Geometry check sheet. Reference: drawing and pictorial views, mm from the part's lowest x, y, z. A direction names the side the tool comes from. Round coordinates to 2 decimals unless told otherwise and drop trailing zeros. Order: outer loops, then holes, each group sorted by start corner. A loop starts at its lowest first (then second) coordinate and runs counter-clockwise, first axis right, second up.
Q1. Depth check by flat-ended pin: P1, Ø1, axis at y = 22.5, z = 12, coming from the -X side; P2, Ø6.5, axis at x = 54, y = 13.5, coming from the -Z side; P3, Ø2.5, axis at x = 25.5, y = 27.5, coming from the +Z side; P4, Ø8, axis at x = 13.5, z = 37.5, coming from the +Y side. Enter the tip coordinate at first touch or a pass-through.
Q2. Mould release check, pull along X, two halves, no side actions. Record for the marked faces 4, 5, 6 and 7: +X half, -X half, draft (parallel to the pull), parting line (faces both ways), or undercut.
Q3. Cross-section at C-C on z = 18. Record the cut outline in (x, y).
Q4. Set-up check for the marked faces 1, 2 and 3: record each of +Z, -Z, +X, -X, +Y, -Y from which the full face is reachable in a straight line by a thin tool's end or side.
Q5. Scan lines: probe 1 along Y at (x, z) = (7, 26.5); probe 2 along Z at (x, y) = (30, 26); probe 3 along X at (y, z) = (6.5, 37.5). Record each from-to range of solid material in increasing order.
Q6. Cross-section at A-A on y = 6. Record the cut outline in (x, z).
Q7. Cross-section at D-D on x = 53. Record the cut outline in (y, z), then the cut area to 3 significant figures.
Q8. Cross-section at B-B on x = 30. Record the cut outline in (y, z), then the cut area to 3 significant figures.
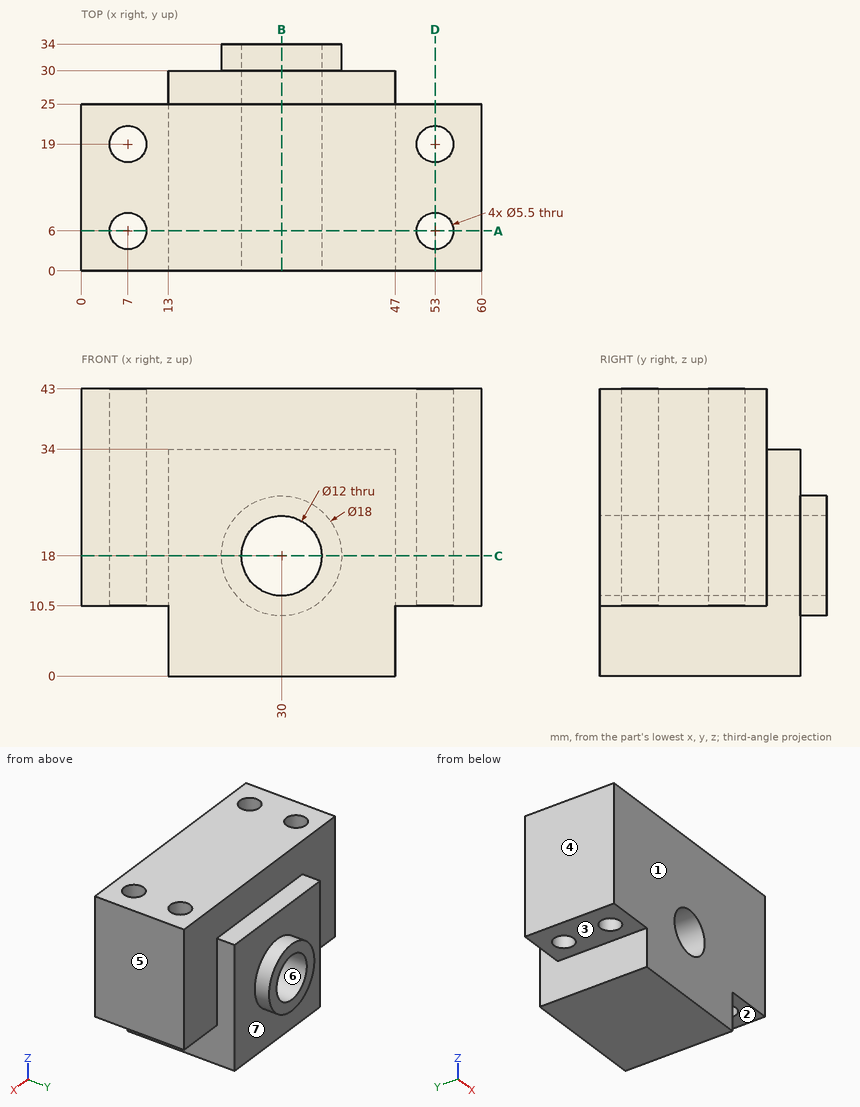
Results found:
1. P1: stops at x = 0
1. P2: stops at z = 10.5
1. P3: stops at z = 34
1. P4: stops at y = 30
2. face 4: -X half
2. face 5: +X half
2. face 6: undercut
2. face 7: draft
3. outline: (0, 0) - (24, 0) - (24, 34) - (21, 34) - (21, 30) - (13, 30) - (13, 25) - (0, 25) - close; (36, 0) - (60, 0) - (60, 25) - (47, 25) - (47, 30) - (39, 30) - (39, 34) - (36, 34) - close; hole circle Ø5.5 at (7, 6); hole circle Ø5.5 at (7, 19); hole circle Ø5.5 at (53, 6); hole circle Ø5.5 at (53, 19)
4. face 1: +Z, -Z, +X, -X, -Y
4. face 2: -Z, +X, +Y, -Y
4. face 3: -Z, -X, +Y, -Y
5. probe 1: y = 0 to 3.25, 8.75 to 16.25, 21.75 to 25
5. probe 2: z = 0 to 12, 24 to 34
5. probe 3: x = 0 to 4.3, 9.7 to 50.3, 55.7 to 60
6. outline: (0, 10.5) - (4.25, 10.5) - (4.25, 43) - (0, 43) - close; (9.75, 10.5) - (13, 10.5) - (13, 0) - (47, 0) - (47, 10.5) - (50.25, 10.5) - (50.25, 43) - (9.75, 43) - close; (55.75, 10.5) - (60, 10.5) - (60, 43) - (55.75, 43) - close; hole circle Ø12 at (30, 18)
7. outline: (0, 10.5) - (3.25, 10.5) - (3.25, 43) - (0, 43) - close; (8.75, 10.5) - (16.25, 10.5) - (16.25, 43) - (8.75, 43) - close; (21.75, 10.5) - (25, 10.5) - (25, 43) - (21.75, 43) - close
7. area: 455 mm2
8. outline: (0, 0) - (30, 0) - (30, 9) - (34, 9) - (34, 12) - (0, 12) - close; (0, 24) - (34, 24) - (34, 27) - (30, 27) - (30, 34) - (25, 34) - (25, 43) - (0, 43) - close
8. area: 909 mm2
